```python
from build123d import *

# Parameters (mm, degrees)
SKETCH1_W           = 161.8
SKETCH1_H           = 124
SKETCH1_R           = 1.65
BOSS_EXTRUDE1_DEPTH = 2


with BuildPart() as part:
    # Sketch1 → Boss-Extrude1 (new body)
    with BuildSketch(Plane(origin=(0, 0, 0), x_dir=(1, 0, 0), z_dir=(0, 1, 0))):
        with Locations((0, 14)):
            Rectangle(SKETCH1_W, SKETCH1_H)
        with Locations((-70.9, 38)):
            Circle(SKETCH1_R, mode=Mode.SUBTRACT)
        with Locations((-70.9, 26)):
            Circle(SKETCH1_R, mode=Mode.SUBTRACT)
        with Locations((-70.9, -26)):
            Circle(SKETCH1_R, mode=Mode.SUBTRACT)
        with Locations((-70.9, -38)):
            Circle(SKETCH1_R, mode=Mode.SUBTRACT)
        with Locations((70.9, 38)):
            Circle(SKETCH1_R, mode=Mode.SUBTRACT)
        with Locations((70.9, 26)):
            Circle(SKETCH1_R, mode=Mode.SUBTRACT)
        with Locations((70.9, -26)):
            Circle(SKETCH1_R, mode=Mode.SUBTRACT)
        with Locations((70.9, -38)):
            Circle(SKETCH1_R, mode=Mode.SUBTRACT)
    extrude(amount=BOSS_EXTRUDE1_DEPTH)


solid = part.part
```
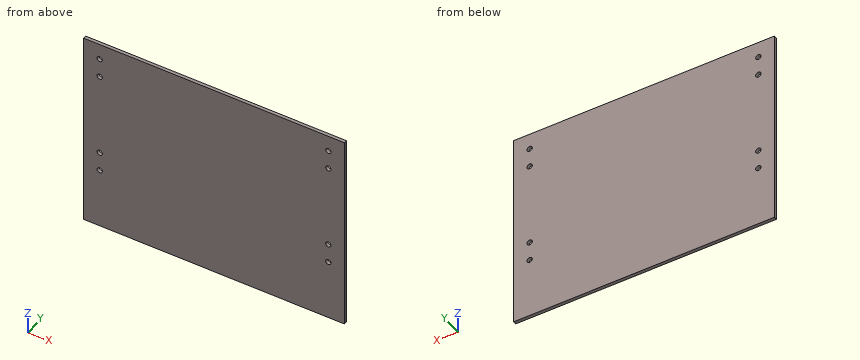
For this review, take the finished solid that the model builds, in its own axes (mm). Coordinates: 2 decimals unless noted, no trailing zeros. Loops run counter-clockwise (first coordinate to the right, second up) from the corner with the lowest first, then second, coordinate; pieces in that order, holes last.
1. For line 1 (Z direction, x = 70.9, y = 1.05); line 2 (X direction, y = 1.5, z = 38), list the stretches that pass through material, from the lowest coordinate up.
2. Add section B-B, the plane x = 70.9. Give the boundary of the cut face in (y, z), then the cut area to 3 significant figures.
3. Add section A-A, the plane z = -38. Give the boundary of the cut face in (x, y).
4. Insertion check: P1, Ø2, axis at x = -70.9, z = 38, coming from the +Y side. The pin has a flat end and moves straight along its axis. Give the tip position at first contact, or say it passes through.
Result:
1. line 1: z = -76 to -39.65, -36.35 to -27.65, -24.35 to 24.35, 27.65 to 36.35, 39.65 to 48
1. line 2: x = -80.9 to -72.55, -69.25 to 69.25, 72.55 to 80.9
2. outline: (0, -76) - (2, -76) - (2, -39.65) - (0, -39.65) - close; (0, -36.35) - (2, -36.35) - (2, -27.65) - (0, -27.65) - close; (0, -24.35) - (2, -24.35) - (2, 24.35) - (0, 24.35) - close; (0, 27.65) - (2, 27.65) - (2, 36.35) - (0, 36.35) - close; (0, 39.65) - (2, 39.65) - (2, 48) - (0, 48) - close
2. area: 222 mm2
3. outline: (-80.9, 0) - (-72.55, 0) - (-72.55, 2) - (-80.9, 2) - close; (-69.25, 0) - (69.25, 0) - (69.25, 2) - (-69.25, 2) - close; (72.55, 0) - (80.9, 0) - (80.9, 2) - (72.55, 2) - close
4. P1: passes through
